from build123d import *

# Parameters (mm, degrees)
SKETCH_1_R      = 1.5
EXTRUDE_1_DEPTH = 2


with BuildPart() as part:
    # 草图1 → 凸台-拉伸1 (new body)
    with BuildSketch(Plane.XY):
        Polygon((3, 3.164176285), (0, 34), (0, 22.228513357), (-3, 3.164176285), (-3, -13.164176285), (3, -13.164176285), align=None)
        Circle(SKETCH_1_R, mode=Mode.SUBTRACT)
        with Locations((0, -10)):
            Circle(SKETCH_1_R, mode=Mode.SUBTRACT)
    extrude(amount=EXTRUDE_1_DEPTH)


solid = part.part
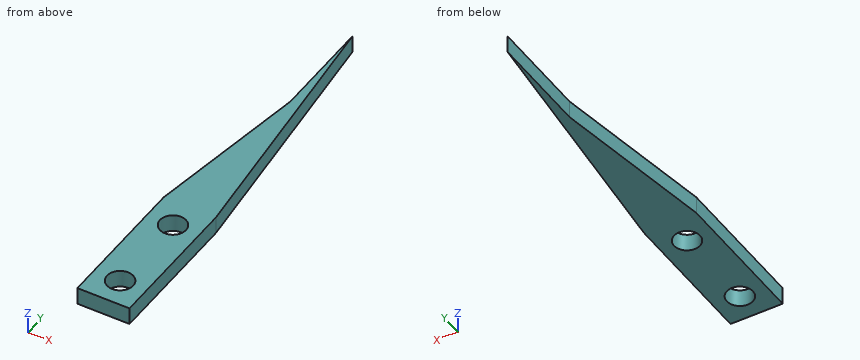
Read the model definition and answer for the solid it produces. Units are mm, in the model's axes. Round coordinates to 2 decimals unless told otherwise and drop trailing zeros. Order: outer loops, then holes, each group sorted by start corner. A loop starts at its lowest first (then second) coordinate and runs counter-clockwise, first axis right, second up.
1) The part is cut by section A-A on z = 0.65. Write down the section's boundary in (x, y).
2) The part is cut by section B-B on y = 0. Write down the section's boundary in (x, z), plus the area to 3 significant figures.
3) The part is cut by section C-C on x = 0.7. Write down the section's boundary in (y, z), plus the area to 3 significant figures.
4) Straight lines are drawn through the part: L1, parallel to X at y = 25, z = 0.7; L2, parallel to X at y = 28, z = 1.3. For each, find the intervals that lie inside material, in ascending order.
5) A flat-ended cylindrical pin translates along its axis: pin 1 (1.8 mm diameter, centred on x = 0, y = 0, fed in from -Z). Find the tip coordinate at first contact, or state that the pin passes through.
6) The part is cut by section D-D on y = 29. Write down the section's boundary in (x, z), plus the area to 3 significant figures.
Resolved:
1. outline: (-3, -13.16) - (3, -13.16) - (3, 3.16) - (0, 34) - (0, 22.23) - (-3, 3.16) - close; hole circle Ø3 at (0, -10); hole circle Ø3 at (0, 0)
2. outline: (-3, 0) - (-1.5, 0) - (-1.5, 2) - (-3, 2) - close; (1.5, 0) - (3, 0) - (3, 2) - (1.5, 2) - close
2. area: 6.00 mm2
3. outline: (-13.16, 0) - (-11.33, 0) - (-11.33, 2) - (-13.16, 2) - close; (-8.67, 0) - (-1.33, 0) - (-1.33, 2) - (-8.67, 2) - close; (1.33, 0) - (26.8, 0) - (26.8, 2) - (1.33, 2) - close
3. area: 69.3 mm2
4. L1: x = 0 to 0.88
4. L2: x = 0 to 0.58
5. pin 1: passes through
6. outline: (0, 0) - (0.49, 0) - (0.49, 2) - (0, 2) - close
6. area: 0.973 mm2
